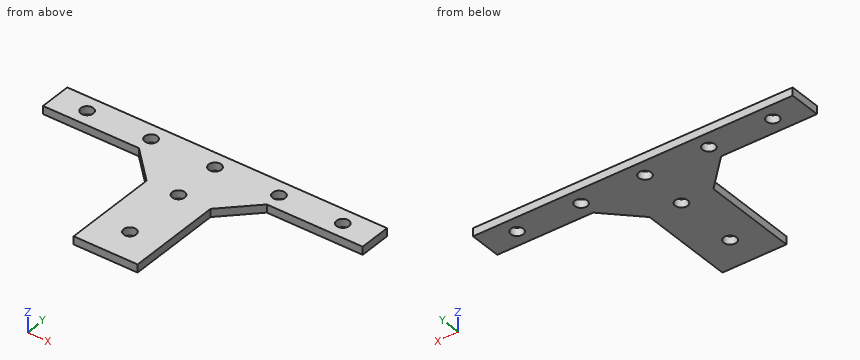
from build123d import *

# Parameters (mm, degrees)
BOSS_EXTRUDE1_DEPTH    = 3.175
F_10_CLEARANCE_HOLE1_D = 4.9784


with BuildPart() as part:
    # Sketch1 → Boss-Extrude1 (new body)
    with BuildSketch(Plane.XY):
        Polygon((41.275, -25.4), (41.275, -63.5), (66.675, -63.5), (66.675, -25.4), (79.375, -12.7), (117.475, -12.7), (117.475, 0), (-9.525, 0), (-9.525, -12.7), (28.575, -12.7), align=None)
    extrude(amount=BOSS_EXTRUDE1_DEPTH)

    # #10 Clearance Hole1 (through all)
    with Locations(Plane.XY.offset(3.175)):
        with Locations((3.175, -6.35), (28.575, -6.35), (53.975, -6.35), (104.775, -6.35), (53.975, -25.4), (53.975, -50.8), (79.375, -6.35)):
            Hole(F_10_CLEARANCE_HOLE1_D / 2)


solid = part.part
Can you work these out from the model? Positions are in its coordinate system, mm. Round coordinates to 2 decimals unless told otherwise and drop trailing zeros. Loops run counter-clockwise (first coordinate to the right, second up) from the corner with the lowest first, then second, coordinate; pieces in that order, holes last. Notation, with made-up numbers: (71.25, 4.5) - (102.25, 4.5) arc R29 ccw to (102.25, 26.5) - close; hole circle Ø9 at (-26.75, -16.5). An arc over 180 degrees is marked (long way). Use CSV: the item, a comma, the result in double quotes. Start each with the question number.
1) Please list where these lines run through material, in increasing order: probe 1 along X at (y, z) = (-8.5, 0.35) (3 decimals); probe 2 along X at (y, z) = (-25.5, 1.4) (3 decimals); probe 3 along X at (y, z) = (-28.5, 1.65) (3 decimals). Write a range as [from, to].
2) For pin 1 Ø1.6 at (y, z) = (-45, 2) entering from +X (3 decimals), with a flat end and sliding along its axis, tell me the tip position at first contact or that it passes through.
3) If we section it at B-B on y = -6.35: Write out the boundary of the cut face in (x, z) (3 decimals).
4) If we section it at D-D on x = -0.5: Write out the boundary of the cut face in (y, z) (3 decimals).
5) If we section it at A-A on y = -50.8: Write out the boundary of the cut face in (x, z) (3 decimals), plus the area to 3 significant figures.
6) If we section it at C-C on z = 1.3: Write out the boundary of the cut face in (x, y) (3 decimals), plus the area to 3 significant figures.
Geometry results:
1,probe 1,"x = [-9.525, 1.921], [4.429, 27.321], [29.829, 52.721], [55.229, 78.121], [80.629, 103.521], [106.029, 117.475]"
1,probe 2,"x = [41.275, 51.488], [56.462, 66.675]"
1,probe 3,"x = [41.275, 66.675]"
2,pin 1,"stops at x = 66.675"
3,outline,"(-9.525, 0) - (0.686, 0) - (0.686, 3.175) - (-9.525, 3.175) - close; (5.664, 0) - (26.086, 0) - (26.086, 3.175) - (5.664, 3.175) - close; (31.064, 0) - (51.486, 0) - (51.486, 3.175) - (31.064, 3.175) - close; (56.464, 0) - (76.886, 0) - (76.886, 3.175) - (56.464, 3.175) - close; (81.864, 0) - (102.286, 0) - (102.286, 3.175) - (81.864, 3.175) - close; (107.264, 0) - (117.475, 0) - (117.475, 3.175) - (107.264, 3.175) - close"
4,outline,"(-12.7, 0) - (0, 0) - (0, 3.175) - (-12.7, 3.175) - close"
5,outline,"(41.275, 0) - (51.486, 0) - (51.486, 3.175) - (41.275, 3.175) - close; (56.464, 0) - (66.675, 0) - (66.675, 3.175) - (56.464, 3.175) - close"
5,area,"64.8 mm2"
6,outline,"(-9.525, -12.7) - (28.575, -12.7) - (41.275, -25.4) - (41.275, -63.5) - (66.675, -63.5) - (66.675, -25.4) - (79.375, -12.7) - (117.475, -12.7) - (117.475, 0) - (-9.525, 0) - close; hole circle Ø4.978 at (3.175, -6.35); hole circle Ø4.978 at (28.575, -6.35); hole circle Ø4.978 at (53.975, -50.8); hole circle Ø4.978 at (53.975, -25.4); hole circle Ø4.978 at (53.975, -6.35); hole circle Ø4.978 at (79.375, -6.35); hole circle Ø4.978 at (104.775, -6.35)"
6,area,"2,930 mm2"
